Geometry: see drawing. Coordinates: mm, zero at the bounding-box minimum. A direction names the side the tool comes from. Round coordinates to 2 decimals unless told otherwise and drop trailing zeros. Loops run counter-clockwise (first coordinate to the right, second up) from the corner with the lowest first, then second, coordinate; pieces in that order, holes last. Notation, with made-up numbers: (-29.75, 61) - (-0.75, 61) arc R24 ccw to (-0.75, 75) - close; hole circle Ø10 at (49, 14.5). An arc over 180 degrees is marked (long way). Write item = value, one per line. Start each with the question number.
Item 1: Section C-C (z = 88). Return loops of the section in (x, y), plus the area to 3 significant figures.
Item 2: Section A-A (y = 30). Return loops of the section in (x, z).
Item 3: First-contact query: pin 1 (4 mm diameter, centred on x = 73, z = 139, fed in from +Y); pin 2 (6 mm diameter, centred on x = 48, y = 26, fed in from +Z); pin 3 (3 mm diameter, centred on x = 94.5, z = 46.5, fed in from +Y). Flat tips, straight axial feed; report the tip coordinate or a pass-through.
Item 4: Line query: line 1 (Z direction, x = 127.5, y = 41.5); line 2 (X direction, y = 31, z = 19). Output: solid intervals per line, ascending. Write a range as from..to.
Item 5: Section B-B (x = 92). Return loops of the section in (y, z), plus the area to 3 significant figures.
Item 6: Section D-D (z = 168.5). Return loops of the section in (x, y).
Item 7: Access query for the marked faces 1, 2 and 3. Directions: +Z, -Z, +X, -X, +Y, -Y. A direction counts if a zero-diameter tool reaches every point of the face in a straight line with its end or side. Return the directions, or none.
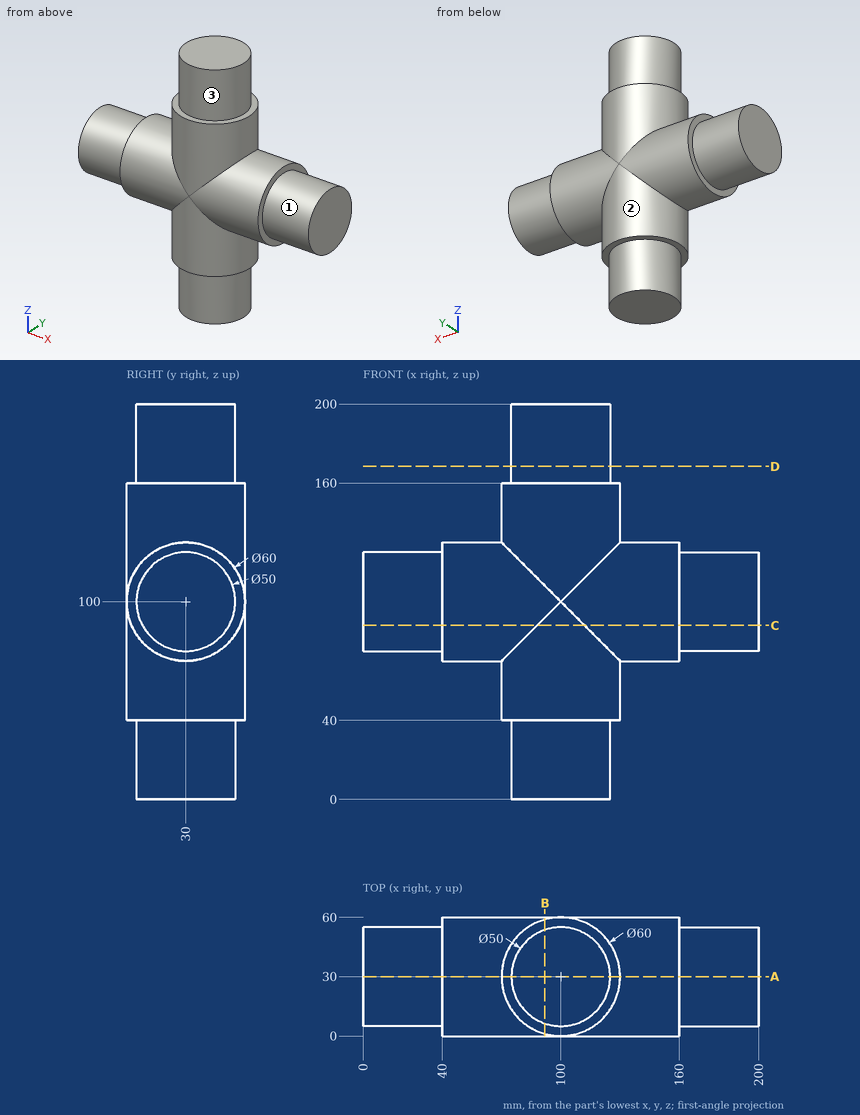
Taken from the geometry:
q1.outline = (0, 8.07) - (40, 8.07) - (40, 2.5) - (88, 2.5) arc R30 ccw to (112, 2.5) - (160, 2.5) - (160, 8.07) - (200, 8.07) - (200, 51.93) - (160, 51.93) - (160, 57.5) - (112, 57.5) arc R30 ccw to (88, 57.5) - (40, 57.5) - (40, 51.93) - (0, 51.93) - close
q1.area = 10,200 mm^2
q2.outline = (0, 75) - (40, 75) - (40, 70) - (70, 70) - (70, 40) - (75, 40) - (75, 0) - (125, 0) - (125, 40) - (130, 40) - (130, 70) - (160, 70) - (160, 75) - (200, 75) - (200, 125) - (160, 125) - (160, 130) - (130, 130) - (130, 160) - (125, 160) - (125, 200) - (75, 200) - (75, 160) - (70, 160) - (70, 130) - (40, 130) - (40, 125) - (0, 125) - close
q3.pin_1 = 46.58
q3.pin_2 = 129.98
q3.pin_3 = 59.73
q4.line_1 = 40..160
q4.line_2 = 75.02..124.98
q5.outline = (1.09, 40) - (6.31, 40) - (6.31, 0) - (53.69, 0) - (53.69, 40) - (58.91, 40) - (58.91, 92) arc R30 ccw to (58.91, 108) - (58.91, 160) - (53.69, 160) - (53.69, 200) - (6.31, 200) - (6.31, 160) - (1.09, 160) - (1.09, 108) arc R30 ccw to (1.09, 92) - close
q5.area = 10,800 mm^2
q6.outline = circle Ø50 at (100, 30)
q7.face_1 = +X
q7.face_2 = -Z
q7.face_3 = +Z
